Could you check a few things on this drawing? It's one solid part, dimensions in mm from its lowest x, y, z. A direction names the side the tool comes from. Coordinates: 2 decimals unless noted, no trailing zeros. Order: outer loops, then holes, each group sorted by start corner. A loop starts at its lowest first (then second) coordinate and runs counter-clockwise, first axis right, second up. Notation, with made-up numbers: M 4,-39.5 L 58,-39.5 A23 ccw 58,-13.5 Z; hole C 28.25,61 d4. An arc over 180 degrees is marked long. Answer as CSV lines item,"result". Start each with the question number.
1. I need wall thicknesses on line 1 along Z through (x, y) = (29.65, 1.5); line 2 along X through (y, z) = (1, 66.81); line 3 along X through (y, z) = (12, 10.5). Which ranges of each line are inside material? Lowest first, please. Write a range as from..to.
2. If we section it at B-B (y = 19.75): List the corners of the cut face in (x, z) for me, plus the area to 3 significant figures.
3. On a 3-axis mill with a long thin cutter (end or side, diameter ignored), from which of +Z, -Z, +X, -X, +Y, -Y can I reach the whole of each face in a straight line? I mean the marked faces 1 and 2. Say none if no direction works.
4. Will these pins go through, and if not, where does the flat tip stop? pin 1 (18 mm diameter, centred on x = 28.5, z = 46, fed in from +Y); pin 2 (1.9 mm diameter, centred on x = 29.65, z = 66.81, fed in from -Y).
5. If we section it at D-D (x = 3): List the corners of the cut face in (y, z) for me, plus the area to 3 significant figures.
6. If we section it at A-A (x = 29.65): List the corners of the cut face in (y, z) for me, plus the area to 3 significant figures.
7. If we section it at C-C (z = 66.81): List the corners of the cut face in (x, y) for me, plus the area to 3 significant figures.
8. If we mould it in two halves opening along X, with no side actions, what happens to the marked faces 3, 4 and 5? For each: released by +X, released by -X, zero draft, split by the parting line, or undercut.
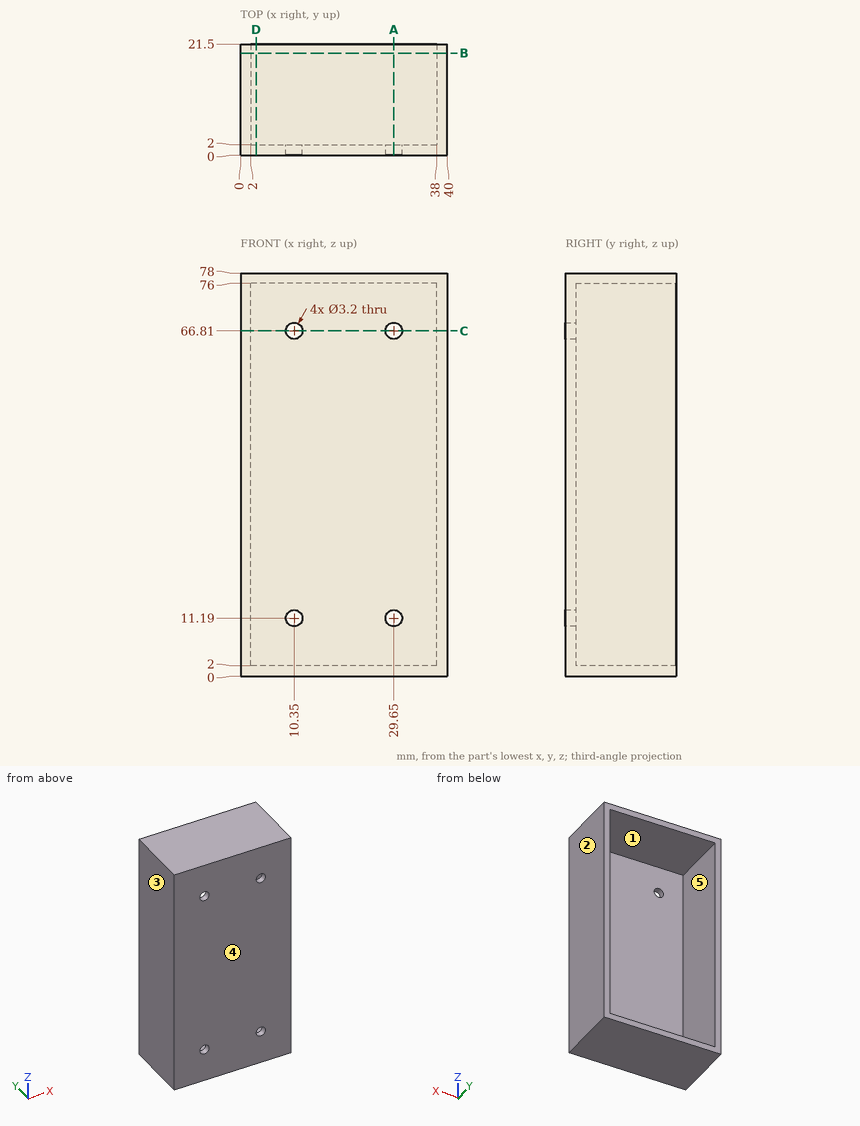
Solved:
1,line 1,"0..9.59, 12.79..65.21, 68.41..78"
1,line 2,"0..8.75, 11.95..28.05, 31.25..40"
1,line 3,"0..2, 38..40"
2,outline,"M 0,0 L 40,0 L 40,78 L 0,78 Z; hole M 2,2 L 38,2 L 38,76 L 2,76 Z"
2,area,"456 mm²"
3,face 1,"+Y"
3,face 2,"+Z, -Z, +X, +Y, -Y"
4,pin 1,"y = 2"
4,pin 2,"through"
5,outline,"M 0,0 L 21.5,0 L 21.5,2 L 2,2 L 2,76 L 21.5,76 L 21.5,78 L 0,78 Z"
5,area,"234 mm²"
6,outline,"M 0,0 L 21.5,0 L 21.5,2 L 2,2 L 2,9.59 L 0,9.59 Z; M 0,12.79 L 2,12.79 L 2,65.21 L 0,65.21 Z; M 0,68.41 L 2,68.41 L 2,76 L 21.5,76 L 21.5,78 L 0,78 Z"
6,area,"221 mm²"
7,outline,"M 0,0 L 8.75,0 L 8.75,2 L 2,2 L 2,21.5 L 0,21.5 Z; M 11.95,0 L 28.05,0 L 28.05,2 L 11.95,2 Z; M 31.25,0 L 40,0 L 40,21.5 L 38,21.5 L 38,2 L 31.25,2 Z"
7,area,"145 mm²"
8,face 3,"released by -X"
8,face 4,"zero draft"
8,face 5,"undercut"
